Input: part model. Units: mm. Frame: model coordinates. A direction names the side the tool comes from. Round coordinates to 2 decimals unless told otherwise and drop trailing zeros. Order: outer loops, then holes, each group sorted by start corner. A loop starts at its lowest first (then second) coordinate and runs counter-clockwise, first axis right, second up.
Item 1: Cut plane B-B on z = 17. Output: boundary loops of the cut face in (x, y), then the cut area to 3 significant figures.
Item 2: Line query: L1, parallel to Z at x = -54, y = 1.5; L2, parallel to Z at x = -4.5, y = 4; L3, parallel to X at y = 1.1, z = -39.5. Output: solid intervals per line, ascending.
Item 3: First-contact query: pin 1 (2.5 mm diameter, centred on x = -58, y = 1.5, fed in from +Z); pin 2 (5 mm diameter, centred on x = 24, z = -34, fed in from -Y); pin 3 (1.5 mm diameter, centred on x = 57, y = 2, fed in from -Z); pin 4 (3 mm diameter, centred on y = 3, z = -11.5, fed in from -X). Flat tips, straight axial feed; report the tip coordinate or a pass-through.
Item 4: Cut plane C-C on x = -15.5. Output: boundary loops of the cut face in (y, z).
Item 5: Reachability of faces 1 (the flat face through (56, 2, -4.5)), 2 (the flat face through (-56, 3, 4.5)), 3 (the flat face through (56, 2, 4.5)) from +Z, -Z, +X, -X, +Y, -Y: full face, straight path, thin tool, end or side. Return the list, or none.
Item 6: Cut plane A-A on y = 1.1. Output: boundary loops of the cut face in (x, z).
```python
from build123d import *

# Parameters (mm, degrees)
SKETCH3_R           = 52.5
BOSS_EXTRUDE1_DEPTH = 5
SKETCH5_W           = 16
SKETCH5_H           = 9
BOSS_EXTRUDE2_DEPTH = 2.5


with BuildPart() as part:
    # Sketch3 → Boss-Extrude1 (new body)
    with BuildSketch(Plane(origin=(0, 0, 0), x_dir=(1, 0, 0), z_dir=(0, 1, 0))):
        with Locations(Location((0, 0, 0), (0, 0, 270))):
            Circle(SKETCH3_R)
    extrude(amount=BOSS_EXTRUDE1_DEPTH)

    # Sketch5 → Boss-Extrude2 (add, symmetric)
    with BuildSketch(Plane(origin=(0, 2.5, 0), x_dir=(1, 0, 0), z_dir=(0, 1, 0))):
        with Locations((52.5, 0)):
            Rectangle(SKETCH5_W, SKETCH5_H)
        with Locations((-52.5, 0)):
            Rectangle(SKETCH5_W, SKETCH5_H)
    extrude(amount=BOSS_EXTRUDE2_DEPTH, both=True)


solid = part.part
```
From the geometry:
1. outline: (-49.67, 0) - (49.67, 0) - (49.67, 5) - (-49.67, 5) - close
1. area: 497 mm2
2. L1: z = -4.5 to 4.5
2. L2: z = -52.31 to 52.31
2. L3: x = -34.58 to 34.58
3. pin 1: stops at z = 4.5
3. pin 2: stops at y = 0
3. pin 3: stops at z = -4.5
3. pin 4: stops at x = -51.54
4. outline: (0, -50.16) - (5, -50.16) - (5, 50.16) - (0, 50.16) - close
5. face 1: -Z, +X, +Y, -Y
5. face 2: +Z, -X, +Y, -Y
5. face 3: +Z, +X, +Y, -Y
6. outline: (-60.5, -4.5) - (-52.31, -4.5) arc R52.5 ccw to (52.31, -4.5) - (60.5, -4.5) - (60.5, 4.5) - (52.31, 4.5) arc R52.5 ccw to (-52.31, 4.5) - (-60.5, 4.5) - close
